Geometry check sheet. Reference: the model listing, model coordinates, mm. Face numbers are marked on the shaded views. A direction names the side the tool comes from. Give positions to 0.01 mm unless a question says otherwise; leave off trailing zeros. Write each loop counter-clockwise with the first axis right and the second up, starting at its lowest first coordinate (ties: lowest second). Pieces come first, ordered by that corner, then holes.
(1) Cross-section at D-D (x = 0). Record the boundary of the cut face in (y, z), and give its area (3 significant figures).
(2) Thickness scan on line 1 along Y through (x, z) = (-48.5, -14.5); line 2 along X through (y, z) = (77, -1); line 3 along Y through (x, z) = (17, 98). Record the ranges inside material, lowest first.
(3) Cross-section at B-B (x = 15.5). Record the boundary of the cut face in (y, z), and give its area (3 significant figures).
(4) Cross-section at A-A (z = 0). Record the boundary of the cut face in (x, y), and give its area (3 significant figures).
(5) Tool access check on the marked faces 1, 2 and 3. Record the directions out of +Z, -Z, +X, -X, +Y, -Y that give a thin tool (end or side, any length) a straight path to the whole face; none if there is none.
(6) Cross-section at C-C (y = 97). Record the boundary of the cut face in (x, z), and give its area (3 significant figures).
(7) Depth check by flat-ended pin: P1, Ø12, axis at x = -20, z = 64.5, coming from the -Y side; P2, Ø2, axis at y = 50.5, z = 26.5, coming from the +X side; P3, Ø12, axis at y = 179.5, z = 4.5, coming from the +X side. Enter the tip coordinate at first touch or a pass-through.
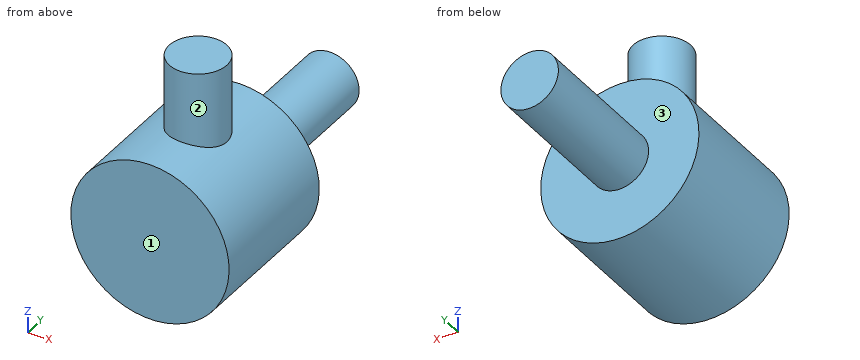
```python
from build123d import *

# Parameters (mm, degrees)
SKETCH1_R                = 55
BOSS_EXTRUDE1_DEPTH      = 100
SKETCH2_R                = 20
BOSS_EXTRUDE2_DEPTH      = 100
BOSS_EXTRUDE3_DEPTH      = 50
BOSS_EXTRUDE3_DEPTH_BACK = 20
SKETCH3_R                = 20


with BuildPart() as part:
    # Sketch1 → Boss-Extrude1 (new body)
    with BuildSketch(Plane(origin=(0, 0, 0), x_dir=(1, 0, 0), z_dir=(0, 1, 0))):
        with Locations(Location((0, 0, 0), (0, 0, 270))):
            Circle(SKETCH1_R)
    extrude(amount=BOSS_EXTRUDE1_DEPTH)

    # Sketch2 → Boss-Extrude2 (add)
    with BuildSketch(Plane(origin=(0, 100, 0), x_dir=(1, 0, 0), z_dir=(0, 1, 0))):
        with Locations(Location((0, 0, 0), (0, 0, 270))):
            Circle(SKETCH2_R)
    extrude(amount=BOSS_EXTRUDE2_DEPTH)

    # Sketch3 → Boss-Extrude3 (add, two sides: drawn at the far end of the back side and taken through both)
    with BuildSketch(Plane.XY.offset(55).offset(-BOSS_EXTRUDE3_DEPTH_BACK)):
        with Locations((2.115721614, 50)):
            Circle(SKETCH3_R)
    extrude(amount=BOSS_EXTRUDE3_DEPTH + BOSS_EXTRUDE3_DEPTH_BACK)


solid = part.part
```
Reply:
1. outline: (0, -55) - (100, -55) - (100, -20) - (200, -20) - (200, 20) - (100, 20) - (100, 55) - (69.89, 55) - (69.89, 105) - (30.11, 105) - (30.11, 55) - (0, 55) - close
1. area: 17,000 mm2
2. line 1: y = 0 to 100
2. line 2: x = -54.99 to 54.99
2. line 3: y = 36.64 to 63.36
3. outline: (0, -52.77) - (100, -52.77) - (100, -12.64) - (200, -12.64) - (200, 12.64) - (100, 12.64) - (100, 52.77) - (64.86, 52.77) - (64.86, 105) - (35.14, 105) - (35.14, 52.77) - (0, 52.77) - close
3. area: 14,600 mm2
4. outline: (-55, 0) - (55, 0) - (55, 100) - (20, 100) - (20, 200) - (-20, 200) - (-20, 100) - (-55, 100) - close
4. area: 15,000 mm2
5. face 1: +Z, -Z, +X, -X, -Y
5. face 2: +Z
5. face 3: +Y
6. outline: circle Ø110 at (0, 0)
6. area: 9,500 mm2
7. P1: stops at y = 38.16
7. P2: stops at x = 48.73
7. P3: stops at x = 20
